```python
from build123d import *

# Parameters (mm, degrees)
SKETCH_1_R         = 10
SKETCH_1_R_2       = 3
EXTRUDE_1_DEPTH    = 2
SKETCH_2_R         = 4
SKETCH_2_R_2       = 3
EXTRUDE_1_2_DEPTH  = 3.5
HOLE_WIZARD_M3_1_D = 2.5
SKETCH_6_W         = 1.3
SKETCH_6_H         = 1.5
EXTRUDE_START      = 1.4
SKETCH_7_R         = 3
EXTRUDE_2_DEPTH    = 1.4


with BuildPart() as part:
    # 草图1 → Extrude 1 (new body)
    with BuildSketch(Plane.XY):
        Circle(SKETCH_1_R)
        Circle(SKETCH_1_R_2, mode=Mode.SUBTRACT)
    extrude(amount=EXTRUDE_1_DEPTH)

    # 草图2 → Extrude 1 2 (add)
    with BuildSketch(Plane.XY.offset(2)):
        Circle(SKETCH_2_R)
        Circle(SKETCH_2_R_2, mode=Mode.SUBTRACT)
    extrude(amount=EXTRUDE_1_2_DEPTH)

    # M3 螺纹孔1 (through all)
    with Locations(Plane(origin=(-7, 0, 2), x_dir=(1, 0, 0), z_dir=(0, 0, 1))):
        with Locations((0, 0), (7, 7), (14, 0), (7, -7)):
            Hole(HOLE_WIZARD_M3_1_D / 2)

    # 草图6 → 旋转1 (revolve)
    with BuildSketch(Plane(origin=(0, 0, 0), x_dir=(0, 0, -1), z_dir=(1, 0, 0))):
        with Locations((-2.05, 2.25)):
            Rectangle(SKETCH_6_W, SKETCH_6_H)
    revolve(axis=Axis((0, 0, 0), (0, 0, 1)))

    # 草图7 → 凸台-拉伸2 (add)
    with BuildSketch(Plane(origin=(0, 0, 1.4), x_dir=(-1, 0, 0), z_dir=(0, 0, -1)).offset(EXTRUDE_START)):
        with Locations(Location((0, 0, 0), (0, 0, 270))):
            Circle(SKETCH_7_R)
    extrude(amount=-EXTRUDE_2_DEPTH)


solid = part.part
```
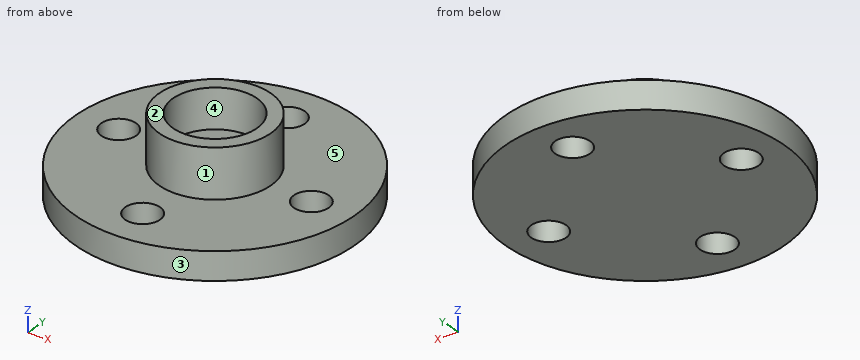
Check sheet for the modelled part. Datum: model origin and axes. Units: mm. Face numbers are marked on the shaded views. A direction names the side the tool comes from. Give positions to 0.01 mm unless a question says otherwise; leave off trailing zeros. Loops run counter-clockwise (first coordinate to the right, second up) from the corner with the lowest first, then second, coordinate; pieces in that order, holes last. Notation, with made-up numbers: (-13, -7.5) - (12, -7.5) arc R22 ccw to (12, 26.5) - close; hole circle Ø8 at (44.5, 76.5). An arc over 180 degrees is marked (long way). One line per question, with ' | ' between items. Start each with the question number.
1. Cross-section at B-B, the plane x = -7.25. Enter the section's corners in (y, z).
2. Draft check along Y on the marked faces 3, 4 and 5. Enter one of: released by +Y, released by -Y, zero draft, split by the parting line, or undercut.
3. Gauge pin test, flat ends, axial feed: pin 1 Ø3 at (x, z) = (2.5, 2) entering from +Y; pin 2 Ø1.8 at (x, y) = (1, -0.5) entering from +Z; pin 3 Ø1.5 at (x, z) = (-6.5, 1) entering from +Y. Record the tip position at first contact, or that the pin passes through.
4. Cross-section at D-D, the plane y = -0.5. Enter the section's corners in (x, z).
5. Material ranges on line 1 along Y through (x, z) = (0, 1.9); line 2 along Y through (x, z) = (0, 3.45); line 3 along Z through (x, y) = (5.5, -1.25), recorded low to high. Write a range as [from, to].
6. Set-up check for the marked faces 1 and 2: record each of +Z, -Z, +X, -X, +Y, -Y from which the full face is reachable in a straight line by a thin tool's end or side.
7. Cross-section at C-C, the plane z = 4.55. Enter the section's corners in (x, y), plus the area to 3 significant figures.
8. Cross-section at A-A, the plane y = 8. Enter the section's corners in (x, z), plus the area to 3 significant figures.
Check result:
1) outline: (-6.89, 0) - (-1.22, 0) - (-1.22, 2) - (-6.89, 2) - close; (1.22, 0) - (6.89, 0) - (6.89, 2) - (1.22, 2) - close
2) face 3: split by the parting line | face 4: undercut | face 5: zero draft
3) pin 1: stops at y = 9.95 | pin 2: stops at z = 2.7 | pin 3: stops at y = 8.18
4) outline: (-9.99, 0) - (-8.15, 0) - (-8.15, 2) - (-9.99, 2) - close; (-5.85, 0) - (5.85, 0) - (5.85, 2) - (3.97, 2) - (3.97, 5.5) - (2.96, 5.5) - (2.96, 2.7) - (1.41, 2.7) - (1.41, 1.4) - (-1.41, 1.4) - (-1.41, 2.7) - (-2.96, 2.7) - (-2.96, 5.5) - (-3.97, 5.5) - (-3.97, 2) - (-5.85, 2) - close; (8.15, 0) - (9.99, 0) - (9.99, 2) - (8.15, 2) - close
5) line 1: y = [-10, -8.25], [-5.75, -1.5], [1.5, 5.75], [8.25, 10] | line 2: y = [-4, -3], [3, 4] | line 3: z = [0, 2]
6) face 1: +Z | face 2: +Z, +X, -X, +Y, -Y
7) outline: circle Ø8 at (0, 0); hole circle Ø6 at (0, 0) | area: 22.0 mm2
8) outline: (-6, 0) - (-0.75, 0) - (-0.75, 2) - (-6, 2) - close; (0.75, 0) - (6, 0) - (6, 2) - (0.75, 2) - close | area: 21.0 mm2
